Model file for the job. Use its own axes, mm. Face numbers are marked on the shaded views. A direction names the side the tool comes from. Round coordinates to 2 decimals unless told otherwise and drop trailing zeros. Loops run counter-clockwise (first coordinate to the right, second up) from the corner with the lowest first, then second, coordinate; pieces in that order, holes last.
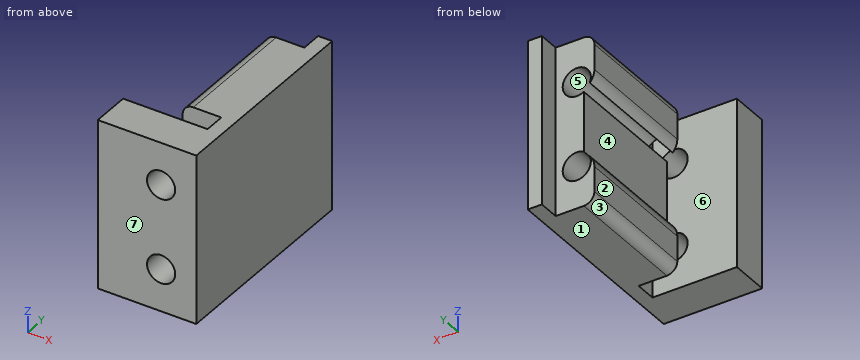
from build123d import *

# Parameters (mm, degrees)
SKETCH1_W           = 12
SKETCH1_H           = 24
BOSS_EXTRUDE1_DEPTH = 5.5
SKETCH2_W           = 2
SKETCH2_H           = 24
BOSS_EXTRUDE2_DEPTH = 29.5
BOSS_EXTRUDE4_START = 3
SKETCH4_W           = 5.5
SKETCH4_H           = 24
BOSS_EXTRUDE4_DEPTH = 18
SKETCH5_W           = 9.25
SKETCH5_H           = 18
CUT_EXTRUDE1_DEPTH  = 1.5
FILLET1_R           = 2.5
SKETCH6_R           = 2
CUT_EXTRUDE2_DEPTH  = 31.170349683
FILLET2_R           = 1.5


with BuildPart() as part:
    # Sketch1 → Boss-Extrude1 (new body)
    with BuildSketch(Plane(origin=(0, 0, 0), x_dir=(1, 0, 0), z_dir=(0, 1, 0))):
        Rectangle(SKETCH1_W, SKETCH1_H)
    extrude(amount=BOSS_EXTRUDE1_DEPTH)

    # Sketch2 → Boss-Extrude2 (add)
    with BuildSketch(Plane(origin=(0, 0, 0), x_dir=(1, 0, 0), z_dir=(0, 1, 0))):
        with Locations((7, 0)):
            Rectangle(SKETCH2_W, SKETCH2_H)
    extrude(amount=BOSS_EXTRUDE2_DEPTH)

    # Sketch4 → Boss-Extrude4 (add)
    with BuildSketch(Plane(origin=(0, 5.5, 0), x_dir=(1, 0, 0), z_dir=(0, 1, 0)).offset(BOSS_EXTRUDE4_START)):
        with Locations((3.25, 0)):
            Rectangle(SKETCH4_W, SKETCH4_H)
    extrude(amount=BOSS_EXTRUDE4_DEPTH)

    # Sketch5 → Cut-Extrude1 (cut)
    with BuildSketch(Plane.ZY.offset(-0.5)):
        with Locations((0, 17.5)):
            Rectangle(SKETCH5_W, SKETCH5_H)
    extrude(amount=-CUT_EXTRUDE1_DEPTH, mode=Mode.SUBTRACT)

    # Fillet1
    # the kernel refuses this fillet: 2.5 mm, written as the material it takes off along each edge
    with BuildSketch(Plane(origin=(0.5, 32.228219619, 4.625), x_dir=(0, 0, 1), z_dir=(0, -1, 0)), Plane(origin=(0.5, 8.5, -4.625), x_dir=(0, 0, -1), z_dir=(0, 1, 0))) as fillet1_piece_1:
        with BuildLine():
            CenterArc((2.291287847, -2.5), FILLET1_R, 90, 66.421821522)
            Line((0, -1.5), (0, 0))
            Line((0, 0), (2.291287847, 0))
        make_face()
    extrude(amount=23.728219619, mode=Mode.SUBTRACT)

    # Sketch6 → Cut-Extrude2 (cut, through all)
    with BuildSketch(Plane(origin=(0, 26.5, 0), x_dir=(1, 0, 0), z_dir=(0, 1, 0))):
        with Locations(Location((3, -6, 0), (0, 0, 270))):
            Circle(SKETCH6_R)
        with Locations(Location((3, 6, 0), (0, 0, 90))):
            Circle(SKETCH6_R)
    extrude(amount=-CUT_EXTRUDE2_DEPTH, mode=Mode.SUBTRACT)

    # Fillet2
    fillet2_edges = [part.edges().sort_by_distance(p)[0] for p in [
        (0.5, 17.5, -12),
        (0.5, 17.5, 12),
    ]]
    fillet(fillet2_edges, radius=FILLET2_R)


solid = part.part
Q1. Slice it at B-B on y = 4.5. Give the cut face in (x, z), plus the area to 3 significant figures.
Q2. Tool access for the marked faces 1, 2, 3 and 4: list every direction of +Z, -Z, +X, -X, +Y, -Y with a clear straight run to the whole face (end or side of a thin tool).
Q3. Flat gauge pins, fed straight in: P1, Ø4.5, axis at y = 17.5, z = -1, coming from the -X side; P2, Ø4.5, axis at x = 3, z = -6, coming from the +Y side; P3, Ø4, axis at y = 9.5, z = -3.5, coming from the -X side; P4, Ø3.5, axis at x = 3, z = -6, coming from the -Y side. Where does each tip first touch, or does it go through?
Q4. Slice it at A-A on x = 3. Give the cut face in (y, z), plus the area to 3 significant figures.
Q5. Slice it at D-D on y = 17. Give the cut face in (x, z).
Q6. Probe line 1 (Y direction, x = 4.5, z = -4.25); line 2 (Z direction, x = 3, y = 14); line 3 (Z direction, x = 4.75, y = 1.5). List the from-to ranges inside material, lowest first.
Q7. Pull direction Y, two halves, no side cores. Call the marked faces 5, 6 and 7: pulls with the +Y half, pulls with the -Y half, needs draft (parallel to the pull), parting line crosses it, or undercut.
Q8. Slice it at C-C on z = -8.75. Give the cut face in (x, y), plus the area to 3 significant figures.
Reply:
1. outline: (-6, -12) - (8, -12) - (8, 12) - (-6, 12) - close; hole circle Ø4 at (3, -6); hole circle Ø4 at (3, 6)
1. area: 311 mm2
2. face 1: -Z, +X, -X, +Y, -Y
2. face 2: +Z, -Z, -X, +Y
2. face 3: -Z, -X, +Y
2. face 4: -X, +Y
3. P1: stops at x = 2
3. P2: stops at y = 26.5
3. P3: stops at x = 0.94
3. P4: passes through
4. outline: (0, -12) - (5.5, -12) - (5.5, -8) - (0, -8) - close; (0, -4) - (5.5, -4) - (5.5, 4) - (0, 4) - close; (0, 8) - (5.5, 8) - (5.5, 12) - (0, 12) - close; (8.5, -12) - (26.5, -12) - (26.5, -8) - (8.5, -8) - close; (8.5, -4) - (26.5, -4) - (26.5, 4) - (8.5, 4) - close; (8.5, 8) - (26.5, 8) - (26.5, 12) - (8.5, 12) - close
4. area: 376 mm2
5. outline: (0.5, -10.5) arc R1.5 ccw to (2, -12) - (8, -12) - (8, 12) - (2, 12) arc R1.5 ccw to (0.5, 10.5) - (0.5, 6.92) arc R2.5 ccw to (1.15, 5.23) arc R2 cw (long way) to (2, 4.27) - (2, -4.27) arc R2 cw (long way) to (1.15, -5.23) arc R2.5 ccw to (0.5, -6.92) - close
6. line 1: y = 0 to 5.5, 8.5 to 26.5
6. line 2: z = -12 to -8, -4 to 4, 8 to 12
6. line 3: z = -12 to -6.97, -5.03 to 5.03, 6.97 to 12
7. face 5: needs draft
7. face 6: undercut
7. face 7: pulls with the -Y half
8. outline: (-6, 0) - (8, 0) - (8, 29.5) - (6, 29.5) - (6, 26.5) - (0.5, 26.5) - (0.5, 8.5) - (6, 8.5) - (6, 5.5) - (-6, 5.5) - close
8. area: 224 mm2
